from build123d import *

# Parameters (mm, degrees)
F0_R     = 7.5
F1_DEPTH = 25
F2_R     = 3
F3_R     = 11
F4_DEPTH = 4


with BuildPart() as f1:
    # F0 (on Front) → F1 (new body)
    with BuildSketch(Plane.XZ):
        with BuildLine():
            Line((100, 50), (-100, 50))
            ThreePointArc((-100, 50), (-114.142136, 44.142136), (-120, 30))
            Line((-120, 30), (-120, -30))
            ThreePointArc((-120, -30), (-114.142136, -44.142136), (-100, -50))
            Line((-100, -50), (100, -50))
            ThreePointArc((100, -50), (114.142136, -44.142136), (120, -30))
            Line((120, -30), (120, 30))
            ThreePointArc((120, 30), (114.142136, 44.142136), (100, 50))
        make_face()
        Circle(F0_R, mode=Mode.SUBTRACT)
    extrude(amount=F1_DEPTH)

    # F2
    f2_edges = [f1.edges().sort_by_distance(p)[0] for p in [
        (0, -25, 50),
        (0, 0, 50),
        (-114.142136, 0, 44.142136),
        (-120, 0, 0),
        (-114.142136, 0, -44.142136),
        (0, 0, -50),
        (114.142136, 0, -44.142136),
        (120, 0, 0),
        (114.142136, 0, 44.142136),
        (-7.5, 0, 0),
    ]]
    fillet(f2_edges, radius=F2_R)

    # F3 (on face) → F4 (cut)
    with BuildSketch(Plane.XZ.offset(25)):
        Circle(F3_R)
    extrude(amount=-F4_DEPTH, mode=Mode.SUBTRACT)


solid = f1.part
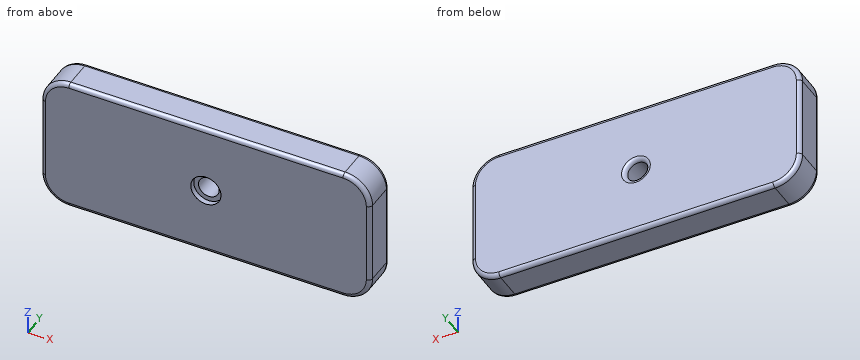
Read the model definition and answer for the solid it produces. Units are mm, in the model's axes. Give positions to 0.01 mm unless a question says otherwise; leave off trailing zeros. Write each loop counter-clockwise with the first axis right and the second up, starting at its lowest first coordinate (ties: lowest second). Pieces come first, ordered by that corner, then holes. Notation, with made-up numbers: (34, 27.5) - (63, 27.5) arc R24 ccw to (63, 40.5) - close; hole circle Ø5 at (-7, 26.25). An arc over 180 degrees is marked (long way). Answer in a Markdown table with one row per item. Add a question column.
Item 1: Section A-A, the plane x = 0 is taken. Write down the section's boundary in (y, z), and give its area (3 significant figures).
Item 2: Section C-C, the plane y = -12.75 is taken. Write down the section's boundary in (x, z), and give its area (3 significant figures).
Item 3: Section B-B, the plane z = 0 is taken. Write down the section's boundary in (x, y).
Item 4: Flat-ended cylindrical pins translate along their axes: P1, Ø13, axis at x = 0, z = 0, coming from the -Y side; P2, Ø17, axis at x = 0, z = 0, coming from the +Y side. Find the tip coordinate at first contact, or state that the pin passes through.
Item 5: Find the intervals of material crossed by L1, parallel to Z at x = 0, y = -22.35; L2, parallel to X at y = -9.75, z = 0; L3, parallel to Z at x = 0, y = -10, in increasing order.
Recorded:
| question | item | result |
|---|---|---|
| 1 | outline | (-25, -47) arc R3 ccw to (-22, -50) - (-3, -50) arc R3 ccw to (0, -47) - (0, -10.5) arc R3 ccw to (-3, -7.5) - (-21, -7.5) - (-21, -11) - (-25, -11) - close; (-25, 11) - (-21, 11) - (-21, 7.5) - (-3, 7.5) arc R3 ccw to (0, 10.5) - (0, 47) arc R3 ccw to (-3, 50) - (-22, 50) arc R3 ccw to (-25, 47) - close |
| 1 | area | 2,090 mm2 |
| 2 | outline | (-120, -30) arc R20 ccw to (-100, -50) - (100, -50) arc R20 ccw to (120, -30) - (120, 30) arc R20 ccw to (100, 50) - (-100, 50) arc R20 ccw to (-120, 30) - close; hole circle Ø15 at (0, 0) |
| 2 | area | 23,500 mm2 |
| 3 | outline | (-120, -22) arc R3 ccw to (-117, -25) - (-11, -25) - (-11, -21) - (-7.5, -21) - (-7.5, -3) arc R3 ccw to (-10.5, 0) - (-117, 0) arc R3 ccw to (-120, -3) - close; (7.5, -21) - (11, -21) - (11, -25) - (117, -25) arc R3 ccw to (120, -22) - (120, -3) arc R3 ccw to (117, 0) - (10.5, 0) arc R3 ccw to (7.5, -3) - close |
| 4 | P1 | passes through |
| 4 | P2 | stops at y = -0.76 |
| 5 | L1 | z = -49.98 to -11, 11 to 49.98 |
| 5 | L2 | x = -120 to -7.5, 7.5 to 120 |
| 5 | L3 | z = -50 to -7.5, 7.5 to 50 |
